Can you work these out from the model? Positions are in its coordinate system, mm. A direction names the side the tool comes from. Coordinates: 2 decimals unless noted, no trailing zeros. Order: outer loops, then holes, each group sorted by start corner. A loop starts at its lowest first (then second) coordinate and runs counter-clockwise, first axis right, second up. Notation, with made-up numbers: (-34, 21.5) - (0, 21.5) arc R14 ccw to (0, 47.5) - close; hole circle Ø3 at (8.5, -0.75). An arc over 180 degrees is marked (long way). Return JSON: item names as keys, results as strings. Group by question number.
1) If I drill on line 1 along Y through (x, z) = (-1, 2.3); line 2 along Y through (x, z) = (2.5, 2.1); line 3 along X through (y, z) = (3, 0.35), over which ranges is the centre line in solid material (lowest first)?
2) Imagine slicing it at C-C (y = 1). Write out the boundary of the cut face in (x, z).
3) If we mould it in two halves opening along X, with no side actions, what happens to faces 1 (the face through (10.78, 1.62, 1.25)), 2 (the face through (10.499, -26.896, 1.252)), 3 (the face through (17, -12, 2.54)), 4 (the face through (-25.4, -13, 1))? For each: pulls with the +X half, pulls with the -X half, needs draft (parallel to the pull), parting line crosses it, or undercut.
4) For pin 1 Ø1.5 at (x, z) = (-16.5, 0.5) entering from -Y; pin 2 Ø1 at (x, z) = (-12.5, 1) entering from +Y, each with a flat end and sliding along its axis, tell me the tip position at first contact or that it passes through.
5) Which directions (+Z, -Z, +X, -X, +Y, -Y) give clear straight access to the entire face, cutting with the end or side of a thin tool? Please do faces 5 (the face through (-13, 0, 1)), 6 (the face through (44.45, -12, 1)), 7 (the face through (-13, -25.4, 1)).
6) Imagine slicing it at B-B (x = -18.5). Write out the boundary of the cut face in (y, z).
7) Imagine slicing it at A-A (z = 1.2). Write out the boundary of the cut face in (x, y) (3 decimals).
Autodesk Inventor part; units mm, degrees
ref_plane "YZ Plane" through (0, 0, 0) normal (1, 0, 0) x (0, 1, 0)
ref_plane "XZ Plane" through (0, 0, 0) normal (0, 1, 0) x (-1, 0, 0)
ref_plane "XY Plane" through (0, 0, 0) normal (0, 0, 1) x (1, 0, 0)
sketch "Sketch1" plane through (0, 0, 0) normal (0, 0, 1) x (1, 0, 0)
  line L0 (-25.4, 0) -> (-25.4, -12.7)
  line L1 (19.05, 8.255) -> (44.45, 8.255)
  line L2 (44.45, 8.255) -> (44.45, -12.7)
  line L3 (0, -25.4) -> (-25.4, -25.4)
  line L4 (-25.4, -25.4) -> (-25.4, -12.7)
  line L5 (19.05, -33.655) -> (44.45, -33.655)
  line L6 (44.45, -33.655) -> (44.45, -12.7)
  line L7 (-25.4, 0) -> (0, 0)
  arc A0 (0, 0) -> (19.05, 8.255) centre (2.4365, 20.4857) ccw
  arc A1 (19.05, -33.655) -> (0, -25.4) centre (2.4389, -45.8801) ccw
  dimension "d2" = 12.7
  dimension "d3" = 25.4
  dimension "d4" = 20.955
  dimension "d5" = 20.955
  dimension "d6" = 20.6248
extrude "Extrusion1" add sketch "Sketch1" along normal blind 2.54
sketch "Sketch2" plane through (0, 0, 2.54) normal (0, 0, 1) x (1, 0, 0)
  line L0 (0, 0) -> (-25.4, 0)
  line L1 (-25.4, 0) -> (-25.4, -25.4)
  line L2 (-25.4, -25.4) -> (0, -25.4)
  arc A0 (19.05, -33.655) -> (0, -25.4) centre (2.4389, -45.8801) ccw
  line L3 (19.05, -33.655) -> (44.45, -33.655)
  line L4 (44.45, -33.655) -> (44.45, 8.255)
  line L5 (44.45, 8.255) -> (19.05, 8.255)
  arc A1 (0, 0) -> (19.05, 8.255) centre (2.4365, 20.4857) ccw
properties part number "Sweep"
Calculated:
{
 "1": {"line 1": "-25.4 to 0", "line 2": "-25.26 to -0.14", "line 3": "13.38 to 44.45"},
 "2": {"outline": "(9.21, 0) - (44.45, 0) - (44.45, 2.54) - (9.21, 2.54) - close"},
 "3": {"face 1": "undercut", "face 2": "undercut", "face 3": "needs draft", "face 4": "pulls with the -X half"},
 "4": {"pin 1": "y = -25.4", "pin 2": "y = 0"},
 "5": {"face 5": "+Z, -Z, -X, +Y", "face 6": "+Z, -Z, +X, +Y, -Y", "face 7": "+Z, -Z, -X, -Y"},
 "6": {"outline": "(-25.4, 0) - (0, 0) - (0, 2.54) - (-25.4, 2.54) - close"},
 "7": {"outline": "(-25.4, -25.4) - (0, -25.4) arc R20.625 cw to (19.05, -33.655) - (44.45, -33.655) - (44.45, 8.255) - (19.05, 8.255) arc R20.63 cw to (0, 0) - (-25.4, 0) - close"}
}
